Source: three-view drawing plus pictorial views. Frame: mm from the lowest corner of the part. Round coordinates to 2 decimals unless told otherwise and drop trailing zeros. Loops run counter-clockwise (first coordinate to the right, second up) from the corner with the lowest first, then second, coordinate; pieces in that order, holes last. Notation, with made-up numbers: (47.5, 22) -> (97.5, 22) arc R32 cw to (97.5, 57) -> close; hole circle Ø9 at (-17.75, -20). An arc over 180 degrees is marked (long way). Answer in a Markdown table with one row per item.
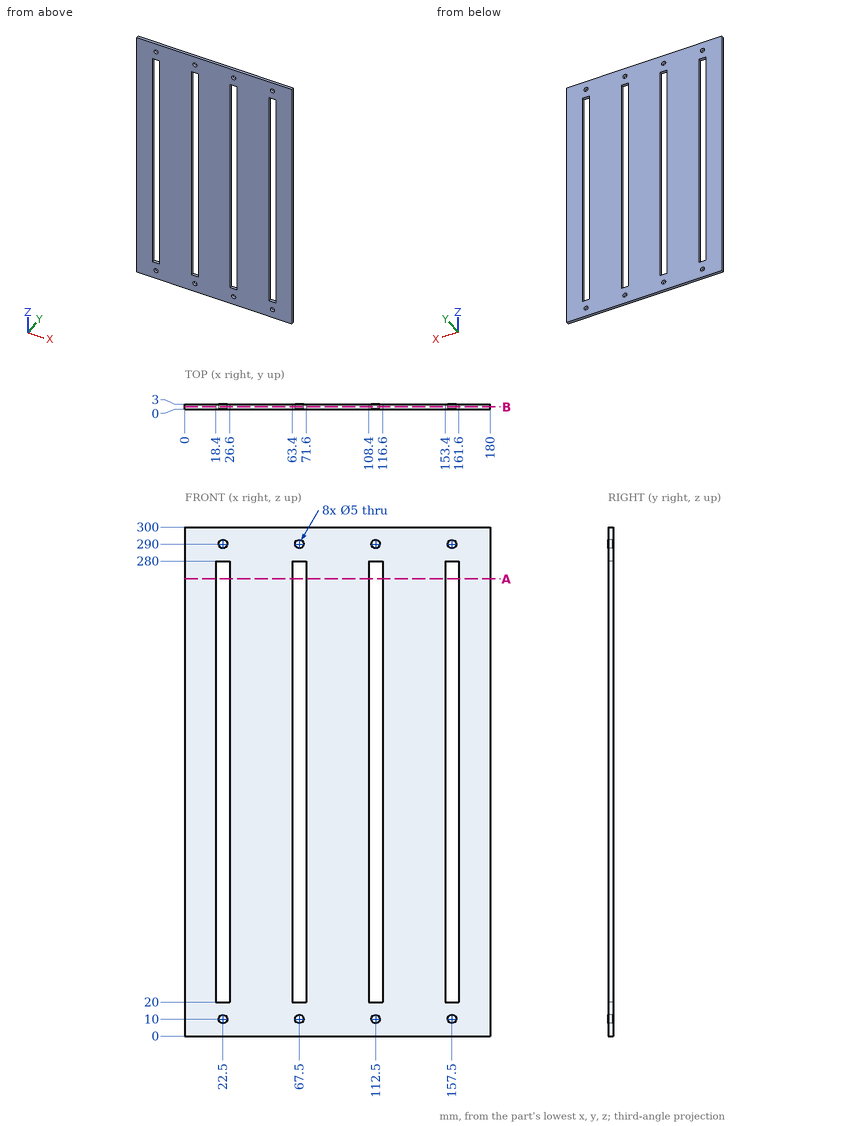
Item 1: Cut plane B-B (y = 1.25). Count the separate pieces of the cut face and the enclosed holes in it, then the cut area to 3 significant figures.
Answer:
| item | result |
|---|---|
| separate pieces | 1 |
| enclosed holes | 12 |
| area | 45,300 mm² |
Item 2: Cut plane A-A (z = 269.5). Output: boundary loops of the cut face in (x, y), then the cut area to 3 significant figures.
Answer:
| item | result |
|---|---|
| outline | (0, 0) -> (18.4, 0) -> (18.4, 3) -> (0, 3) -> close; (26.6, 0) -> (63.4, 0) -> (63.4, 3) -> (26.6, 3) -> close; (71.6, 0) -> (108.4, 0) -> (108.4, 3) -> (71.6, 3) -> close; (116.6, 0) -> (153.4, 0) -> (153.4, 3) -> (116.6, 3) -> close; (161.6, 0) -> (180, 0) -> (180, 3) -> (161.6, 3) -> close |
| area | 442 mm² |
Item 3: Line query: probe 1 along X at (y, z) = (1.3, 290); probe 2 along X at (y, z) = (2.85, 131); probe 3 along Z at (x, y) = (157.5, 1.6). Output: solid intervals per line, ascending. Write a range as [from, to].
Answer:
| item | result |
|---|---|
| probe 1 | x = [0, 20], [25, 65], [70, 110], [115, 155], [160, 180] |
| probe 2 | x = [0, 18.4], [26.6, 63.4], [71.6, 108.4], [116.6, 153.4], [161.6, 180] |
| probe 3 | z = [0, 7.5], [12.5, 20], [280, 287.5], [292.5, 300] |
